Geometry check sheet. Reference: drawing and pictorial views, mm from the part's lowest x, y, z. Give positions to 0.01 mm unless a question says otherwise; leave off trailing zeros. Order: outer loops, then holes, each group sorted by start corner. A loop starts at its lowest first (then second) coordinate and runs counter-clockwise, first axis right, second up. Notation, with made-up numbers: (56, -33.5) -> (61, -33.5) arc R30 ccw to (61, -5.5) -> close; hole circle Ø9 at (6.25, 66). An arc over 180 degrees is marked (long way). Write each question's results on one line, items separated by ' | '.
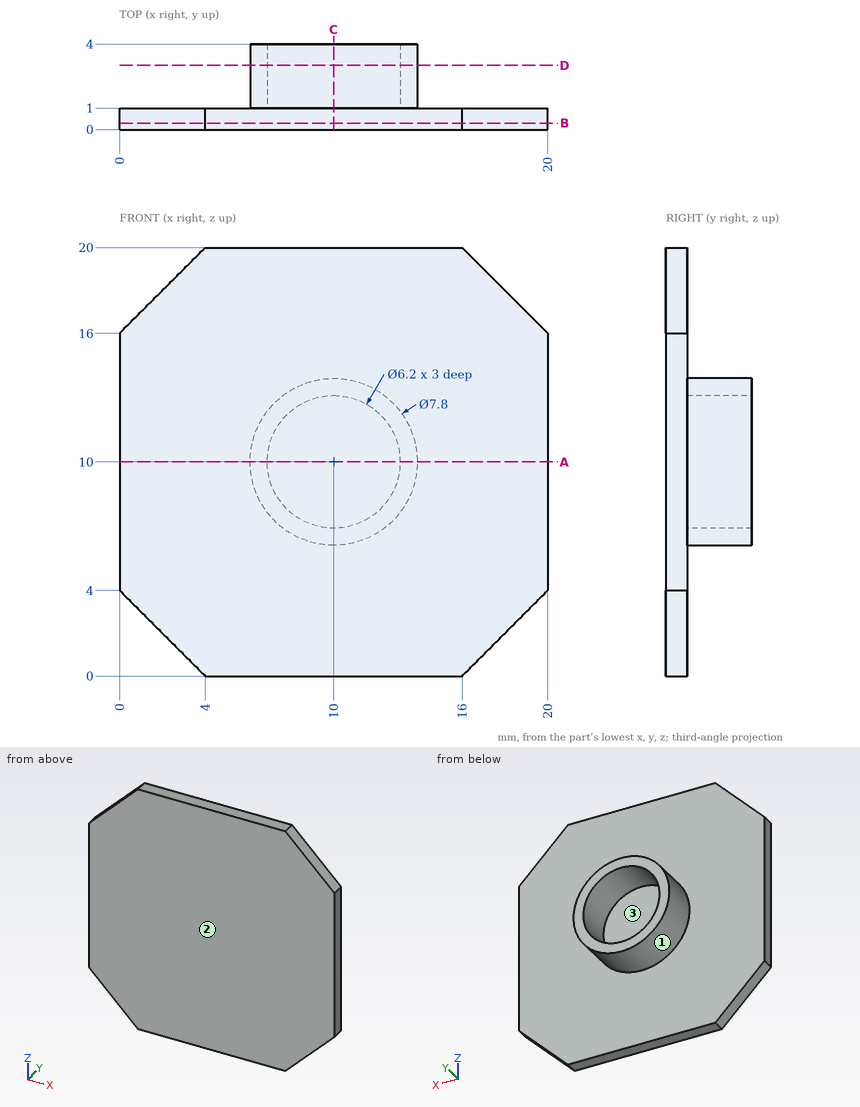
1. Section check B-B on y = 0.3. Record the cut outline in (x, z), then the cut area to 3 significant figures.
Verdict:
outline: (0, 4) -> (4, 0) -> (16, 0) -> (20, 4) -> (20, 16) -> (16, 20) -> (4, 20) -> (0, 16) -> close | area: 368 mm^2
2. Section check C-C on x = 10. Record the cut outline in (y, z).
Verdict:
outline: (0, 0) -> (1, 0) -> (1, 6.1) -> (4, 6.1) -> (4, 6.9) -> (1, 6.9) -> (1, 13.1) -> (4, 13.1) -> (4, 13.9) -> (1, 13.9) -> (1, 20) -> (0, 20) -> close
3. Mould release check, pull along X, two halves, no side actions. Record for the marked faces 1, 2 and 3: +X half, -X half, draft (parallel to the pull), parting line (faces both ways), or undercut.
Verdict:
face 1: parting line | face 2: draft | face 3: undercut
4. Material ranges on probe 1 along X at (y, z) = (2.6, 10); probe 2 along Y at (x, z) = (4.5, 17.25); probe 3 along Z at (x, y) = (11, 3.8), recorded low to high. Write a range as from..to.
Verdict:
probe 1: x = 6.1..6.9, 13.1..13.9 | probe 2: y = 0..1 | probe 3: z = 6.23..7.07, 12.93..13.77
5. Gauge pin test, flat ends, axial feed: pin 1 Ø1 at (y, z) = (3.5, 15.5) entering from +X; pin 2 Ø8 at (x, z) = (8, 18) entering from +Y. Record the tip position at first contact, or that the pin passes through.
Verdict:
pin 1: passes through | pin 2: stops at y = 1
6. Section check D-D on y = 3. Record the cut outline in (x, z), then the cut area to 3 significant figures.
Verdict:
outline: circle Ø7.8 at (10, 10); hole circle Ø6.2 at (10, 10) | area: 17.6 mm^2
7. Section check A-A on z = 10. Record the cut outline in (x, y), then the cut area to 3 significant figures.
Verdict:
outline: (0, 0) -> (20, 0) -> (20, 1) -> (13.9, 1) -> (13.9, 4) -> (13.1, 4) -> (13.1, 1) -> (6.9, 1) -> (6.9, 4) -> (6.1, 4) -> (6.1, 1) -> (0, 1) -> close | area: 24.8 mm^2
